Job drawing, mm, ordinate dimensions from the low corner. One solid piece. Give positions to 0.01 mm unless a question says otherwise; leave off trailing zeros. Order: outer loops, then holes, each group sorted by start corner. A loop starts at its lowest first (then second) coordinate and runs counter-clockwise, first axis right, second up.
1. Slice it at C-C on x = 10. List the corners of the cut face in (y, z).
2. Mould opens along Z. For the marked faces 1, 2 and 3 say: +Z half, -Z half, draft (parallel to the pull), parting line (faces both ways), or undercut.
3. Slice it at D-D on x = 15. List the corners of the cut face in (y, z), and give its area (3 significant figures).
4. Slice it at B-B on y = 1.95. List the corners of the cut face in (x, z).
5. Slice it at A-A on z = 18. List the corners of the cut face in (x, y), and give its area (3 significant figures).
6. Probe line 1 (X direction, y = 2.35, z = 10); line 2 (Z direction, x = 9.5, y = 2.1); line 3 (X direction, y = 0.65, z = 10). List the from-to ranges inside material, lowest first.
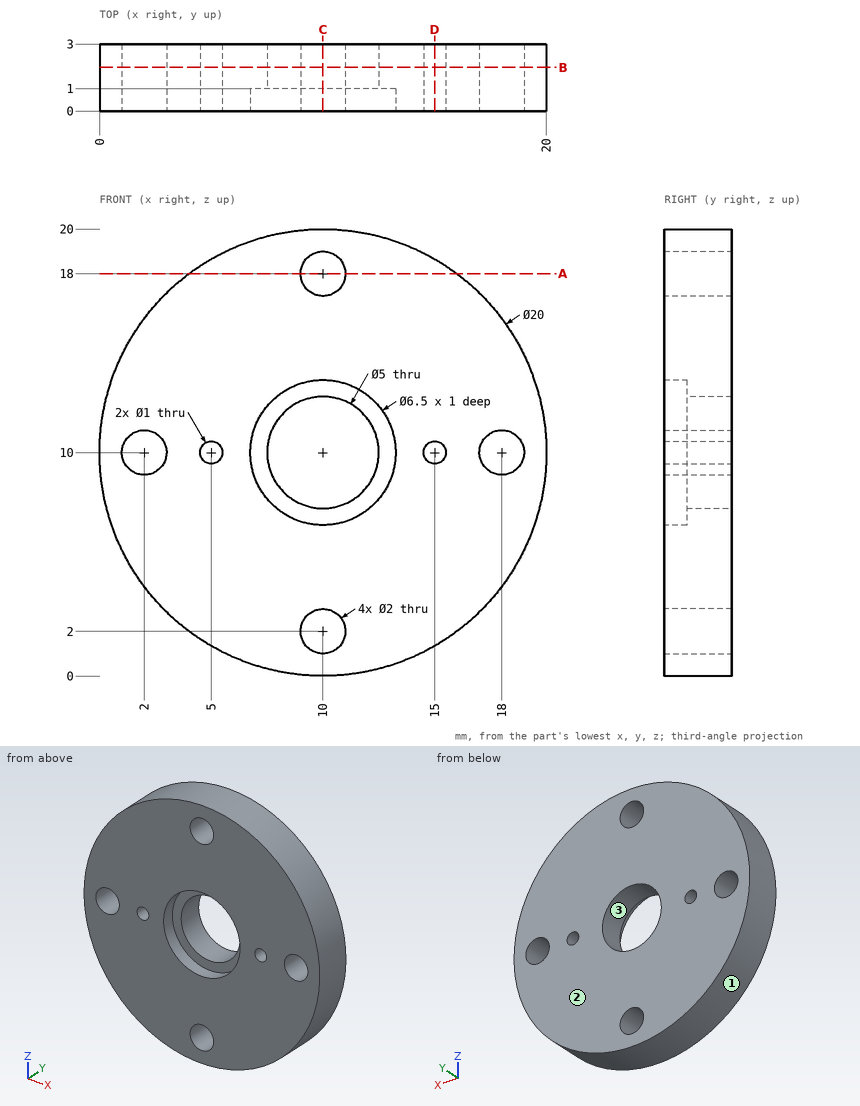
Data:
1. outline: (0, 0) - (3, 0) - (3, 1) - (0, 1) - close; (0, 3) - (3, 3) - (3, 7.5) - (1, 7.5) - (1, 6.75) - (0, 6.75) - close; (0, 13.25) - (1, 13.25) - (1, 12.5) - (3, 12.5) - (3, 17) - (0, 17) - close; (0, 19) - (3, 19) - (3, 20) - (0, 20) - close
2. face 1: parting line
2. face 2: draft
2. face 3: undercut
3. outline: (0, 1.34) - (3, 1.34) - (3, 9.5) - (0, 9.5) - close; (0, 10.5) - (3, 10.5) - (3, 18.66) - (0, 18.66) - close
3. area: 49.0 mm2
4. outline: circle Ø20 at (10, 10); hole circle Ø2 at (2, 10); hole circle Ø1 at (5, 10); hole circle Ø5 at (10, 10); hole circle Ø2 at (10, 2); hole circle Ø2 at (10, 18); hole circle Ø1 at (15, 10); hole circle Ø2 at (18, 10)
5. outline: (4, 0) - (9, 0) - (9, 3) - (4, 3) - close; (11, 0) - (16, 0) - (16, 3) - (11, 3) - close
5. area: 30.0 mm2
6. line 1: x = 0 to 1, 3 to 4.5, 5.5 to 7.5, 12.5 to 14.5, 15.5 to 17, 19 to 20
6. line 2: z = 0.01 to 1.13, 2.87 to 7.55, 12.45 to 17.13, 18.87 to 19.99
6. line 3: x = 0 to 1, 3 to 4.5, 5.5 to 6.75, 13.25 to 14.5, 15.5 to 17, 19 to 20
